Can you work these out from the model? Positions are in its coordinate system, mm. A direction names the side the tool comes from. Round coordinates to 2 decimals unless told otherwise and drop trailing zeros. Loops run counter-clockwise (first coordinate to the right, second up) from the corner with the lowest first, then second, coordinate; pieces in that order, holes last. Notation, with made-up numbers: (24.25, 34.5) -> (33.25, 34.5) arc R31 ccw to (33.25, 71.5) -> close; hole circle Ø11 at (-28.75, 75.5). An arc over 180 degrees is marked (long way). Answer as a JSON object with one key per item and string values.
```python
from build123d import *

# Parameters (mm, degrees)
F0_R      = 7.157093
F1_DEPTH  = 25.4
F2_R      = 5.08
F1_FACE_R = 2.077093
F3_DEPTH  = 3.81


with BuildPart() as f1:
    # F0 (on Front) → F1 (new body)
    with BuildSketch(Plane.XZ):
        with Locations((-65.163344, 43.465324)):
            Circle(F0_R)
    extrude(amount=F1_DEPTH)

    # F2
    f2_edges = [f1.edges().sort_by_distance(p)[0] for p in [
        (-72.320437, -25.4, 43.465324),
        (-72.320437, 0, 43.465324),
    ]]
    fillet(f2_edges, radius=F2_R)

    # F1_face (on face) → F3 (join)
    with BuildSketch(Plane(origin=(-65.163344, -25.4, 43.465324), x_dir=(1, 0, 0), z_dir=(0, -1, 0))):
        Circle(F1_FACE_R)
    extrude(amount=F3_DEPTH)


solid = f1.part
```
Q1. If I drill on L1, parallel to Y at x = -66, z = 38.75; L2, parallel to Z at x = -61.25, y = -16.5; L3, parallel to Y at x = -66.25, z = 46.5, over which ranges is the centre line in solid material (lowest first)? Write a range as [from, to].
Determined:
{"L1": "[-24.62, -0.78]", "L2": "[37.47, 49.46]", "L3": "[-25.27, -0.13]"}
Q2. I'm going to push flat-ended pins straight in: pin 1 (2 mm diameter, centred on x = -66, z = 48.5, fed in from +Y); pin 2 (3 mm diameter, centred on y = -7, z = 41.5, fed in from +X); pin 3 (4 mm diameter, centred on x = -70, y = -21, fed in from -Z). Where does each tip first touch, or does it pass through?
Determined:
{"pin 1": "y = -0.42", "pin 2": "x = -58.02", "pin 3": "z = 36.92"}
Q3. On a 3-axis mill with a long thin cutter (end or side, diameter ignored), from which of +Z, -Z, +X, -X, +Y, -Y can I reach the whole of each face in a straight line? I mean faces 1 (the cylindrical face through (-63.245, -27.278, 42.67)), 2 (the cylindrical face through (-61.316, -12.593, 49.5)). Say none if no direction works.
Determined:
{"face 1": "-Y", "face 2": "+Y, -Y"}
Q4. I want a section at A-A, the plane y = -13.75. Write out the boundary of the cut face in (x, z).
Determined:
{"outline": "circle Ø14.31 at (-65.16, 43.47)"}
